Part model, mm, in its own coordinate system. Face numbers are marked on the shaded views. A direction names the side the tool comes from. Coordinates: 2 decimals unless noted, no trailing zeros. Write each loop counter-clockwise with the first axis right and the second up, starting at its lowest first coordinate (ties: lowest second). Pieces come first, ordered by that corner, then holes. Notation, with made-up numbers: (84, 63) - (128, 63) arc R9 cw to (128, 67) - close; hole circle Ø7 at (67, 58). An arc over 180 degrees is marked (long way). Use a Markdown table: item, result.
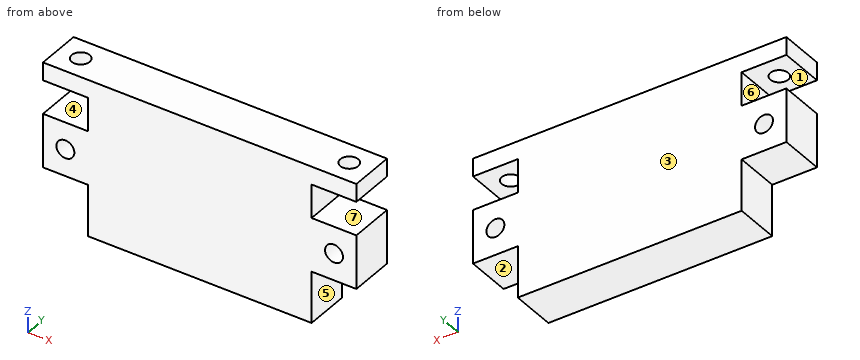
Autodesk Inventor part; units mm, degrees
ref_plane "YZ Plane" through (0, 0, 0) normal (1, 0, 0) x (0, 1, 0)
ref_plane "XZ Plane" through (0, 0, 0) normal (0, 1, 0) x (-1, 0, 0)
ref_plane "XY Plane" through (0, 0, 0) normal (0, 0, 1) x (1, 0, 0)
sketch "Sketch1" plane through (0, 0, 0) normal (0, 1, 0) x (-1, 0, 0)
  line L0 (0, 0) -> (-50, 0)
  line L1 (-50, 0) -> (-50, 35)
  line L2 (-50, 35) -> (0, 35)
  line L3 (0, 35) -> (0, 0)
  line L4 (0, 23.5) -> (10, 23.5)
  line L5 (10, 23.5) -> (10, 11.5)
  line L6 (10, 11.5) -> (0, 11.5)
  line L7 (0, 11.5) -> (0, 23.5)
  line L8 (-50, 23.5) -> (-60, 23.5)
  line L9 (-60, 23.5) -> (-60, 11.5)
  line L10 (-60, 11.5) -> (-50, 11.5)
  line L11 (-50, 11.5) -> (-50, 23.5)
  circle A0 centre (5, 17.5) radius 2
  circle A1 centre (-55, 17.5) radius 2
  dimension "d0" = 50
  dimension "d1" = 35
  dimension "d2" = 10
  dimension "d3" = 12
  dimension "d4" = 11.5
  dimension "d5" = 10
  dimension "d6" = 4
  dimension "d7" = 4
extrude "Extrusion1" add sketch "Sketch1" along normal blind 10
sketch "Sketch2" plane through (0, 0, 35) normal (0, 0, 1) x (1, 0, 0)
  line L0 (50, 0) -> (0, 0)
  line L1 (50, 0) -> (50, 10)
  line L2 (0, 10) -> (50, 10)
  line L3 (0, 0) -> (0, 10)
  line L4 (0, 0) -> (-10, 0)
  line L5 (0, 0) -> (0, 10)
  line L6 (-10, 10) -> (0, 10)
  line L7 (-10, 0) -> (-10, 10)
  line L8 (50, 0) -> (60, 0)
  line L9 (60, 0) -> (60, 10)
  line L10 (50, 10) -> (60, 10)
  line L11 (50, 0) -> (50, 10)
  circle A0 centre (-5, 5) radius 2
  circle A1 centre (55, 5) radius 2
  dimension "d10" = 4
  dimension "d11" = 4
extrude "Extrusion2" add sketch "Sketch2" against normal blind 4
properties part number "00_laserdriver_Pcb"
Item 1: Which spindle directions (+Z, -Z, +X, -X, +Y, -Y) get a long thin tool onto all of the face, cutting with end or side? Do the marked faces 5, 6 and 7. Say none if no direction does.
From the geometry:
| item | result |
|---|---|
| face 5 | -Z, +X, +Y, -Y |
| face 6 | -X, +Y, -Y |
| face 7 | +X, +Y, -Y |
Item 2: Drop flat-ended pins along their axis: P1, Ø3, axis at x = 55, y = 5, coming from the -Z side; P2, Ø1.5, axis at y = 4, z = 28.5, coming from the -X side. Give the stop position or say it passes through.
From the geometry:
| item | result |
|---|---|
| P1 | z = 11.5 |
| P2 | x = 0 |
Item 3: Band-saw the part on B-B, the plane z = 17.5. Give the cut face in (x, y), then the cut area to 3 significant figures.
From the geometry:
| item | result |
|---|---|
| outline | (-10, 0) - (-7, 0) - (-7, 10) - (-10, 10) - close; (-3, 0) - (53, 0) - (53, 10) - (-3, 10) - close; (57, 0) - (60, 0) - (60, 10) - (57, 10) - close |
| area | 620 mm^2 |
Item 4: Band-saw the part on A-A, the plane y = 5. Give the cut face in (x, z), then the cut area to 3 significant figures.
From the geometry:
| item | result |
|---|---|
| outline | (-10, 11.5) - (0, 11.5) - (0, 0) - (50, 0) - (50, 11.5) - (60, 11.5) - (60, 23.5) - (50, 23.5) - (50, 31) - (53, 31) - (53, 35) - (-3, 35) - (-3, 31) - (0, 31) - (0, 23.5) - (-10, 23.5) - close; (-10, 31) - (-7, 31) - (-7, 35) - (-10, 35) - close; (57, 31) - (60, 31) - (60, 35) - (57, 35) - close; hole circle Ø4 at (-5, 17.5); hole circle Ø4 at (55, 17.5) |
| area | 2,010 mm^2 |
Item 5: Band-saw the part on C-C, the plane x = 55. Give the cut face in (y, z), then the cut area to 3 significant figures.
From the geometry:
| item | result |
|---|---|
| outline | (0, 11.5) - (10, 11.5) - (10, 15.5) - (0, 15.5) - close; (0, 19.5) - (10, 19.5) - (10, 23.5) - (0, 23.5) - close; (0, 31) - (3, 31) - (3, 35) - (0, 35) - close; (7, 31) - (10, 31) - (10, 35) - (7, 35) - close |
| area | 104 mm^2 |
Item 6: Two-plate mould, pull along Z, no slides. Class the marked faces 1, 2, 3 and 4: pulls with the +Z half, pulls with the -Z half, needs draft (parallel to the pull), parting line crosses it, or undercut.
From the geometry:
| item | result |
|---|---|
| face 1 | undercut |
| face 2 | pulls with the -Z half |
| face 3 | needs draft |
| face 4 | undercut |
Item 7: Band-saw the part on D-D, the plane z = 32. Give the cut face in (x, y), then the cut area to 3 significant figures.
From the geometry:
| item | result |
|---|---|
| outline | (-10, 0) - (60, 0) - (60, 10) - (-10, 10) - close; hole circle Ø4 at (-5, 5); hole circle Ø4 at (55, 5) |
| area | 675 mm^2 |
Item 8: Drill centre lines: probe 1 along Y at (x, z) = (-5, 33); probe 2 along Z at (x, y) = (51, 2.25); probe 3 along X at (y, z) = (1, 18). Where is each one in solid material? Low to high.
From the geometry:
| item | result |
|---|---|
| probe 1 | 0 to 3, 7 to 10 |
| probe 2 | 11.5 to 23.5, 31 to 35 |
| probe 3 | -10 to -6.94, -3.06 to 53.06, 56.94 to 60 |
